Check sheet for the modelled part. Datum: model origin and axes. Units: mm. A direction names the side the tool comes from. Coordinates: 2 decimals unless noted, no trailing zeros. One line per item, written item: value. Start each with the question number.
1) Gauge pin test, flat ends, axial feed: P1, Ø3, axis at x = -0.5, z = 0, coming from the -Y side; P2, Ø1, axis at y = -22, z = -8.5, coming from the +X side. Record the tip position at first contact, or that the pin passes through.
2) Draft check along Y on faces 3 (the flat face through (0, -10, 12.7)), 4 (the flat face through (0, -13, 12.192)), 5 (the flat face through (3, -25.4, 0)). Enter one of: +Y half, -Y half, draft (parallel to the pull), parting line (faces both ways), or undercut.
3) Set-up check for faces 1 (the flat face through (12.192, -4, 1)), 2 (the flat face through (0, -13, -12.7)): record each of +Z, -Z, +X, -X, +Y, -Y from which the full face is reachable in a straight line by a thin tool's end or side.
4) Scan lines: line 1 along Z through (x, y) = (2.25, -14); line 2 along Y through (x, z) = (7, -7). Record each from-to range of solid material in increasing order. Write a range as [from, to].
```python
from build123d import *

# Parameters (mm, degrees)
F0_W     = 25.4
F0_H     = 25.4
F1_DEPTH = 25.4
F2_R     = 2.54
F3_DEPTH = 0.508
F3_TAPER = -30
F4_R     = 2.54
F5_DEPTH = 0.508
F5_TAPER = -30
F6_R     = 2.54
F7_DEPTH = 0.508
F7_TAPER = -30


with BuildPart() as f1:
    # F0 (on Front) → F1 (new body)
    with BuildSketch(Plane.XZ):
        Rectangle(F0_W, F0_H)
    extrude(amount=F1_DEPTH)

    # F2 (on face) → F3 (cut)
    with BuildSketch(Plane.XY.offset(12.7)):
        with Locations((0, -13.1861664227)):
            Circle(F2_R)
    extrude(amount=-F3_DEPTH, taper=F3_TAPER, mode=Mode.SUBTRACT)

    # F4 (on face) → F5 (cut)
    with BuildSketch(Plane.XZ.offset(25.4)):
        with Locations((-7.8587181904, 7.7246704255)):
            Circle(F4_R)
        Circle(F4_R)
        with Locations((7.2844922543, -7.8815827146)):
            Circle(F4_R)
    extrude(amount=-F5_DEPTH, taper=F5_TAPER, mode=Mode.SUBTRACT)

    # F6 (on face) → F7 (cut)
    with BuildSketch(Plane.YZ.offset(12.7)):
        with Locations((-21.4310005392, 9.2354966214)):
            Circle(F6_R)
        with Locations((-21.3517151213, 0.6695195233)):
            Circle(F6_R)
        with Locations((-21.0309289396, -8.0545796081)):
            Circle(F6_R)
        with Locations((-4.4544605161, 9.4443410787)):
            Circle(F6_R)
        with Locations((-4.3751750982, 0.8783639806)):
            Circle(F6_R)
        with Locations((-4.0543889164, -7.8457351509)):
            Circle(F6_R)
    extrude(amount=-F7_DEPTH, taper=F7_TAPER, mode=Mode.SUBTRACT)


solid = f1.part
```
Answers:
1. P1: stops at y = -24.89
1. P2: stops at x = 12.19
2. face 3: draft
2. face 4: undercut
2. face 5: -Y half
3. face 1: none
3. face 2: -Z, +X, -X, +Y, -Y
4. line 1: z = [-12.7, 12.19]
4. line 2: y = [-24.89, 0]
